Geometry check sheet. Reference: the model listing, model coordinates, mm. A direction names the side the tool comes from. Round coordinates to 2 decimals unless told otherwise and drop trailing zeros.
(1) Set-up check for faces 5 (the face through (-336, 111, -81.184)), 6 (the face through (-44.45, 16.54, -36.42)), 7 (the face through (-330, 37.017, -43)), 8 (the face through (-219.385, 73.407, -40.69)): record each of +Z, -Z, +X, -X, +Y, -Y from which the full face is reachable in a straight line by a thin tool's end or side.
(2) Go/stop test with flat-tipped pins: pin 1 (3 mm diameter, centred on x = -153, y = 46.5, fed in from +Z); pin 2 (10 mm diameter, centred on x = -226, y = 37.5, fed in from +Z); pin 3 (1.5 mm diameter, centred on x = -337.5, y = 35, fed in from +Z); pin 4 (8 mm diameter, centred on x = -102, z = -4.5, fed in from +Y). Record where each tip stops, or that it passes through.
(3) Release check for a two-part mould opening along Y. For faces 1 (the face through (-126.29, 62.26, -39.45)), 2 (the face through (-211.517, 104, -43)), 3 (the face through (-271, 152, -6.128)), 4 (the face through (-172, 0, -39)) record: +Y half, -Y half, draft (parallel to the pull), parting line (faces both ways), or undercut.
(4) Material ranges on line 1 along X through (y, z) = (110, -21); line 2 along Z through (x, y) = (-357, 45.5); line 3 along X through (y, z) = (97, -54), recorded low to high.
from build123d import *

# Parameters (mm, degrees)
SKETCH1_W                       = 800
SKETCH1_H                       = 160
BOSS_EXTRUDE1_DEPTH             = 200
SKETCH2_OUTSIDE_W               = 970
SKETCH2_OUTSIDE_H               = 370
CUT_EXTRUDE1_DEPTH              = 210
CUT_EXTRUDE2_DEPTH              = 210
CUT_EXTRUDE3_DEPTH              = 210
CUT_EXTRUDE14_DEPTH             = 180.8
CUT_EXTRUDE16_DEPTH             = 180.8
CUT_EXTRUDE16_DEPTH_BACK        = 190.8
CUT_EXTRUDE17_DEPTH             = 180.8
CUT_EXTRUDE17_DEPTH_BACK        = 200.8
CUT_EXTRUDE18_REACH             = 184.191
CUT_EXTRUDE18_DIRECTION_2_DEPTH = 200.8


with BuildPart() as part:
    # Sketch1 → Boss-Extrude1 (new body)
    with BuildSketch(Plane(origin=(0, 0, 0), x_dir=(1, 0, 0), z_dir=(0, 1, 0))):
        with Locations((3.854228083, 38.328115975)):
            Rectangle(SKETCH1_W, SKETCH1_H)
    extrude(amount=BOSS_EXTRUDE1_DEPTH)

    # Sketch2 outside → Cut-Extrude1 (cut)
    with BuildSketch(Plane.XY.offset(41.671884025)):
        with Locations((3.854, 100)):
            Rectangle(SKETCH2_OUTSIDE_W, SKETCH2_OUTSIDE_H)
        with BuildLine():
            Line((-376.145771917, 0), (-396.145771917, 105))
            add(Edge.make_bspline(
                [(-396.145771917, 105), (-328.42203974, 170.31399873), (-238.298025694, 200)],
                knots=[0, 0, 0, 1, 1, 1], degree=2))
            Line((-238.298025694, 200), (-202.15321923, 182.191355743))
            Line((-202.15321923, 182.191355743), (-166.597046862, 136.842847328))
            Line((-166.597046862, 136.842847328), (-150.145771917, 65))
            Line((-150.145771917, 65), (-30.145771917, 51.22406477))
            Line((-30.145771917, 51.22406477), (403.854228083, 25.4))
            Line((403.854228083, 25.4), (403.854228083, 0))
            Line((403.854228083, 0), (-376.145771917, 0))
        make_face(mode=Mode.SUBTRACT)
        with BuildLine():
            Line((-211.516960473, 125.283414587), (-211.516960473, 81.582332534))
            Line((-211.516960473, 81.582332534), (-227.477293515, 65))
            Line((-227.477293515, 65), (-359.671028655, 65))
            add(Edge.make_bspline(
                [(-359.671028655, 65), (-375.120725506, 73.239634223), (-363.895142009, 87.176595106)],
                knots=[0, 0, 0, 1, 1, 1], degree=2))
            add(Edge.make_bspline(
                [(-363.895142009, 87.176595106), (-314.715420644, 126.327972018), (-259.142586364, 155.895579394)],
                knots=[0, 0, 0, 1, 1, 1], degree=2))
            add(Edge.make_bspline(
                [(-259.142586364, 155.895579394), (-219.458098431, 165.381218899), (-211.516960473, 125.283414587)],
                knots=[0, 0, 0, 1, 1, 1], degree=2))
        make_face()
    extrude(amount=-CUT_EXTRUDE1_DEPTH, mode=Mode.SUBTRACT)

    # Sketch4 → Cut-Extrude2 (cut)
    with BuildSketch(Plane.XY.offset(41.671884025)):
        Polygon((-277.956260832, 37.01669692), (-383.196571331, 37.01669692), (-376.145771917, 0), (-221.599064851, 0), (-221.599064851, 18.403654878), align=None)
        Polygon((-120.544782401, 18.403654878), (-120.544782401, 0), (-30.906390802, 0), (-30.906390802, 14.724864973), (-58.3780519, 18.403654878), align=None)
    extrude(amount=-CUT_EXTRUDE2_DEPTH, mode=Mode.SUBTRACT)

    # Sketch5 → Cut-Extrude3 (cut)
    with BuildSketch(Plane.XY.offset(41.671884025)):
        Polygon((-30.906390802, 14.724864973), (403.854228083, 0), (-30.906390802, 0), align=None)
    extrude(amount=-CUT_EXTRUDE3_DEPTH, mode=Mode.SUBTRACT)

    # Sketch18 → Cut-Extrude14 (cut)
    with BuildSketch(Plane.XY.offset(41.671884025)):
        Polygon((-30.145771917, 39.610669398), (-30.906390802, 14.724864973), (428.920649615, -48.757692213), (545.595043402, 67.916701575), (-30.145771917, 67.916701575), align=None)
    extrude(amount=-CUT_EXTRUDE14_DEPTH, mode=Mode.SUBTRACT)

    # Sketch19 → Cut-Extrude16 (cut, two sides)
    with BuildSketch(Plane(origin=(0, 182.191355743, 0), x_dir=(1, 0, 0), z_dir=(0, 1, 0))) as cut_extrude16_sk:
        with BuildLine():
            add(Edge.make_bspline(
                [(-238.298025694, 6.128115975), (-213.192031563, -32.648304069), (-166.597046862, -41.671884025)],
                knots=[0, 0, 0, 1, 1, 1], degree=2))
            Line((-238.298025694, 6.128115975), (-396.145771917, 6.128115975))
            Line((-396.145771917, 6.128115975), (-396.145771917, -41.671884025))
            Line((-396.145771917, -41.671884025), (-166.597046862, -41.671884025))
        make_face()
        with BuildLine():
            Line((-30.145771917, -41.671884025), (-30.145771917, 6.128115975))
            add(Edge.make_bspline(
                [(-166.597046862, -41.671884025), (-91.130359602, -37.325806898), (-30.145771917, 6.128115975)],
                knots=[0, 0, 0, 1, 1, 1], degree=2))
            Line((-166.597046862, -41.671884025), (-30.145771917, -41.671884025))
        make_face()
    extrude(amount=CUT_EXTRUDE16_DEPTH, mode=Mode.SUBTRACT)
    extrude(cut_extrude16_sk.sketch, amount=-CUT_EXTRUDE16_DEPTH_BACK, mode=Mode.SUBTRACT)

    # Sketch20 → Cut-Extrude17 (cut, two sides)
    with BuildSketch(Plane(origin=(0, 182.191355743, 0), x_dir=(1, 0, 0), z_dir=(0, 1, 0))) as cut_extrude17_sk:
        with BuildLine():
            Line((-396.145771917, 81.183828909), (-238.298025694, 81.183828909))
            add(Edge.make_bspline(
                [(-168.378508208, 118.328115975), (-205.831679422, 117.897349331), (-238.298025694, 81.183828909)],
                knots=[0.306582709, 0.306582709, 0.306582709, 1, 1, 1], degree=2))
            Line((-168.378508208, 118.328115975), (-396.145771917, 118.328115975))
            Line((-396.145771917, 118.328115975), (-396.145771917, 81.183828909))
        make_face()
        with BuildLine():
            Line((-134.285105115, 111.616416024), (-30.145771917, 76.028115975))
            Line((-30.145771917, 76.028115975), (-30.145771917, 118.328115975))
            Line((-30.145771917, 118.328115975), (-166.597046862, 118.328115975))
            add(Edge.make_bspline(
                [(-134.285105115, 111.616416024), (-150.877544313, 118.147888346), (-166.597046862, 118.328115975)],
                knots=[0, 0, 0, 0.290117528, 0.290117528, 0.290117528], degree=2))
        make_face()
    extrude(amount=CUT_EXTRUDE17_DEPTH, mode=Mode.SUBTRACT)
    extrude(cut_extrude17_sk.sketch, amount=-CUT_EXTRUDE17_DEPTH_BACK, mode=Mode.SUBTRACT)

    # Cut-Extrude18: up to this face of the body (flat: up to its plane)
    cut_extrude18_end = Plane(part.part.faces().sort_by_distance((-97.398178535, 58.94460475, -36.613004679))[0])
    # Sketch21 → Cut-Extrude18 (cut, up to the picked face)
    with BuildSketch(Plane(origin=(0, 182.191355743, 0), x_dir=(1, 0, 0), z_dir=(0, 1, 0)), mode=Mode.PRIVATE) as cut_extrude18_sk1:
        Polygon((-238.298025694, 81.183828909), (-30.145771917, 76.028115975), (-30.145771917, 124.841771597), (-244.744601957, 124.841771597), align=None)
    cut_extrude18_tool1 = split(extrude(cut_extrude18_sk1.sketch, amount=-CUT_EXTRUDE18_REACH, mode=Mode.PRIVATE), bisect_by=cut_extrude18_end, keep=Keep.BOTH, mode=Mode.PRIVATE)
    add(cut_extrude18_tool1.solids().sort_by_distance((-133.846358, 182.191356, -101.823698))[0], mode=Mode.SUBTRACT)
    # Sketch21 → Cut-Extrude18 (cut, up to the picked face)
    with BuildSketch(Plane(origin=(0, 182.191355743, 0), x_dir=(1, 0, 0), z_dir=(0, 1, 0)), mode=Mode.PRIVATE) as cut_extrude18_sk2:
        Polygon((-238.298025694, 6.128115975), (-30.145771917, 6.128115975), (-30.145771917, -32.297232434), (-30.145771917, -55.493942553), (-238.298025694, -55.493942553), align=None)
    cut_extrude18_tool2 = split(extrude(cut_extrude18_sk2.sketch, amount=-CUT_EXTRUDE18_REACH, mode=Mode.PRIVATE), bisect_by=cut_extrude18_end, keep=Keep.BOTH, mode=Mode.PRIVATE)
    add(cut_extrude18_tool2.solids().sort_by_distance((-134.221899, 182.191356, 24.682913))[0], mode=Mode.SUBTRACT)

    # Sketch21 → Cut-Extrude18 direction 2 (cut)
    with BuildSketch(Plane(origin=(0, 182.191355743, 0), x_dir=(1, 0, 0), z_dir=(0, 1, 0))):
        Polygon((-238.298025694, 81.183828909), (-30.145771917, 76.028115975), (-30.145771917, 124.841771597), (-244.744601957, 124.841771597), align=None)
        Polygon((-238.298025694, 6.128115975), (-30.145771917, 6.128115975), (-30.145771917, -32.297232434), (-30.145771917, -55.493942553), (-238.298025694, -55.493942553), align=None)
    extrude(amount=CUT_EXTRUDE18_DIRECTION_2_DEPTH, mode=Mode.SUBTRACT)


solid = part.part
Answer below:
1. face 5: -Z, -X, +Y, -Y
1. face 6: +Z, -Z, -Y
1. face 7: +Z, -Z, -X, -Y
1. face 8: +Z, -Z
2. pin 1: stops at z = 40.71
2. pin 2: stops at z = 14.74
2. pin 3: passes through
2. pin 4: stops at y = 59.93
3. face 1: +Y half
3. face 2: undercut
3. face 3: draft
3. face 4: -Y half
4. line 1: x = -390.87 to -333.54, -211.52 to -160.45
4. line 2: z = -81.18 to -6.13
4. line 3: x = -394.62 to -351.26, -211.52 to -157.47
